Check sheet for the modelled part. Datum: model origin and axes. Units: mm. Face numbers are marked on the shaded views. Give positions to 0.01 mm unless a question says otherwise; leave off trailing zeros. Order: outer loops, then holes, each group sorted by start corner. A loop starts at its lowest first (then second) coordinate and runs counter-clockwise, first axis right, second up.
Item 1: Sectioned sample at B-B on y = 1.25. Record the boundary of the cut face in (x, z).
Item 2: Material ranges on line 1 along X through (y, z) = (1.95, 0); line 2 along Z through (x, y) = (0, 0.2), recorded low to high.
Item 3: Gauge pin test, flat ends, axial feed: P1, Ø3, axis at x = -0.5, z = -1.5, coming from the -Y side; P2, Ø1.8, axis at x = -0.5, z = -1.5, coming from the +Y side; P3, Ø2, axis at y = 1, z = -11, coming from the +X side. Record the tip position at first contact, or that the pin passes through.
Item 4: Release check for a two-part mould opening along Z. For the marked faces 1, 2 and 3 record: released by +Z, released by -Z, zero draft, split by the parting line, or undercut.
Item 5: Sectioned sample at A-A on y = -2.25. Record the boundary of the cut face in (x, z).
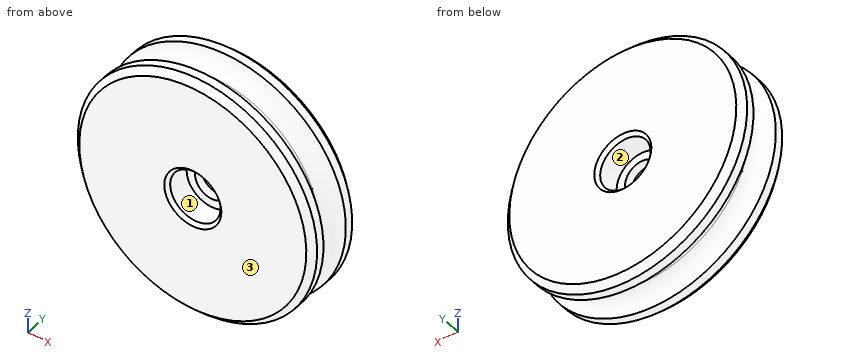
from build123d import *

# Parameters (mm, degrees)
CHAMFER1_SIZE = 0.4


with BuildPart() as part:
    # Sketch1 → Revolve1 (revolve)
    with BuildSketch(Plane(origin=(0, 0, 0), x_dir=(0, 0, -1), z_dir=(1, 0, 0))):
        with BuildLine():
            Line((-3, 3.5), (-13.5274, 3.5))
            Line((-13.5274, 3.5), (-14.2621, 2.7653))
            Line((-14.2621, 2.7653), (-14.2621, 1.7653))
            ThreePointArc((-14.2621, 1.7653), (-13.013844399, 1.248255601), (-12.4968, 0))
            Line((-12.4968, 0), (-2, 0))
            Line((-2, 0), (-2, 0.5))
            Line((-2, 0.5), (-3, 0.5))
            Line((-3, 0.5), (-3, 3.5))
        make_face()
    revolve1 = revolve(axis=Axis((0, 19.017402143, 0), (0, -1, 0)))

    # Mirror1: Revolve1 across plane
    add(revolve1.mirror(Plane.ZX))

    # Chamfer1
    chamfer1_edges = [part.edges().sort_by_distance(p)[0] for p in [
        (0, 3.5, -3),
        (0, -3.5, -3),
    ]]
    chamfer(chamfer1_edges, length=CHAMFER1_SIZE)


solid = part.part
Report:
1. outline: circle Ø26.03 at (0, 0); hole circle Ø6 at (0, 0)
2. line 1: x = -14.26 to -3, 3 to 14.26
2. line 2: z = -12.51 to -2, 2 to 12.51
3. P1: stops at y = -3.18
3. P2: stops at y = 0.5
3. P3: stops at x = 9.81
4. face 1: undercut
4. face 2: undercut
4. face 3: zero draft
5. outline: circle Ø28.52 at (0, 0); hole circle Ø6 at (0, 0)
